The model under review builds one solid part; all positions refer to its coordinate system, in mm. A direction names the side the tool comes from. Round coordinates to 2 decimals unless told otherwise and drop trailing zeros. Loops run counter-clockwise (first coordinate to the right, second up) from the corner with the lowest first, then second, coordinate; pieces in that order, holes last. Notation, with made-up numbers: (31, 13) -> (39, 13) arc R32 ccw to (39, 45) -> close; hole circle Ø5 at (69.5, -14.75). An arc over 180 degrees is marked (long way). Write each question's results on one line, items separated by ' | '. Start each with the question number.
Item 1: We need section B-B (y = -12). Give the boundary of the cut face in (x, z), and give its area (3 significant figures).
Item 2: Clearance check with flat-ended pins moving along their axes: pin 1 Ø4 at (x, y) = (-13.5, -5) entering from +Z; pin 2 Ø5 at (y, z) = (-11.5, 12.5) entering from +X; pin 3 Ø6 at (x, y) = (-21.5, -3) entering from -Z; pin 4 Ø7.5 at (y, z) = (-6.5, 10.5) entering from -X. State where each tip first meets the part, or that it passes through.
Item 3: For L1, parallel to Y at x = 26.5, z = 4.8; L2, parallel to Z at x = 23.5, y = -4.25; L3, parallel to Y at x = -24, z = 4, list the stretches that pass through material, from the lowest coordinate up. Write a range as from..to.
Item 4: Tool access review of faces 1 (the flat face through (22.8, -7.1, 6)), 2 (the flat face through (0, -14.5, 10)): name each direction out of +Z, -Z, +X, -X, +Y, -Y from which nothing blocks a thin tool from reaching the whole face with its end or side.
Item 5: Mouldability with a two-part tool opening along Y and no side actions: class faces 3 (the cylindrical face through (23.267, -8.591, 2.958)), 4 (the flat face through (0, -7, 0)), 5 (the flat face through (0, 0, 10)) as pulls with the +Y half, pulls with the -Y half, needs draft (parallel to the pull), parting line crosses it, or undercut.
Item 6: We need section A-A (y = -7.25). Give the boundary of the cut face in (x, z), and give its area (3 significant figures).
Item 7: We need section D-D (z = 20). Give the boundary of the cut face in (x, y).
Item 8: We need section C-C (x = -26.5). Give the boundary of the cut face in (y, z).
from build123d import *

# Parameters (mm, degrees)
F1_DEPTH = 14.5
F3_DEPTH = 14.5
F4_R     = 1
F5_R     = 3.5
F6_DEPTH = 6


with BuildPart() as f1:
    # F0 (on Front) → F1 (new body)
    with BuildSketch(Plane.XZ):
        with BuildLine():
            Line((-33.5, 0), (-0.8672476206, 0))
            Line((-0.8672476206, 0), (0, 0))
            Line((0, 0), (0.8527118365, 0))
            Line((0.8527118365, 0), (33.5, 0))
            Line((33.5, 0), (33.5, 6))
            Line((33.5, 6), (17.4809702634, 6))
            Line((17.4809702634, 6), (17.4809702634, 16.8373537033))
            Line((17.4809702634, 16.8373537033), (17.4809702634, 18.120359887))
            ThreePointArc((17.4809702634, 18.120359887), (-0.8075640242, 34.9605479634), (-17.4809702634, 16.5198336275))
            Line((-17.4809702634, 16.5198336275), (-17.4809702634, 6))
            Line((-17.4809702634, 6), (-33.5, 6))
            Line((-33.5, 6), (-33.5, 0))
        make_face()
    extrude(amount=F1_DEPTH)

    # F2 (on face) → F3 (cut, through all)
    with BuildSketch(Plane.XZ.offset(14.5)):
        with BuildLine():
            ThreePointArc((0, 23), (-5, 18), (0, 13))
            Line((0, 13), (0, 23))
        make_face()
        with BuildLine():
            Line((0, 23), (0, 13))
            ThreePointArc((0, 13), (3.5355339059, 14.4644660941), (5, 18))
            ThreePointArc((5, 18), (3.5355339059, 21.5355339059), (0, 23))
        make_face()
    extrude(amount=-F3_DEPTH, mode=Mode.SUBTRACT)

    # F4
    f4_edges = [f1.edges().sort_by_distance(p)[0] for p in [
        (-17.48097, -7.25, 6),
        (17.48097, -7.25, 6),
    ]]
    fillet(f4_edges, radius=F4_R)

    # F5 (on face) → F6 (cut, through all)
    with BuildSketch(Plane(origin=(0, 0, 0), x_dir=(1, 0, 0), z_dir=(0, 0, -1))):
        with BuildLine():
            Line((23, 7.25), (30, 7.25))
            ThreePointArc((30, 7.25), (26.5, 10.75), (23, 7.25))
        make_face()
        with BuildLine():
            ThreePointArc((23, 7.25), (26.5, 3.75), (30, 7.25))
            Line((30, 7.25), (23, 7.25))
        make_face()
        with Locations((-26.5, 7.25)):
            Circle(F5_R)
    extrude(amount=-F6_DEPTH, mode=Mode.SUBTRACT)


solid = f1.part
Here are the results:
1) outline: (-33.5, 0) -> (33.5, 0) -> (33.5, 6) -> (18.48, 6) arc R1 cw to (17.48, 7) -> (17.48, 18.12) arc R17.5 ccw (long way) to (-17.48, 16.52) -> (-17.48, 7) arc R1 cw to (-18.48, 6) -> (-33.5, 6) -> close; hole circle Ø10 at (0, 18) | area: 1,210 mm2
2) pin 1: stops at z = 30.68 | pin 2: stops at x = 17.48 | pin 3: stops at z = 0 | pin 4: stops at x = -17.51
3) L1: y = -14.5..-10.75, -3.75..0 | L2: z = 0..6 | L3: y = -14.5..-9.7, -4.8..0
4) face 1: +Z, +X, +Y, -Y | face 2: +Z, -Z, +X, -X, -Y
5) face 3: undercut | face 4: needs draft | face 5: pulls with the +Y half
6) outline: (-33.5, 0) -> (-30, 0) -> (-30, 6) -> (-33.5, 6) -> close; (-23, 0) -> (23, 0) -> (23, 6) -> (18.48, 6) arc R1 cw to (17.48, 7) -> (17.48, 18.12) arc R17.5 ccw (long way) to (-17.48, 16.52) -> (-17.48, 7) arc R1 cw to (-18.48, 6) -> (-23, 6) -> close; (30, 0) -> (33.5, 0) -> (33.5, 6) -> (30, 6) -> close; hole circle Ø10 at (0, 18) | area: 1,120 mm2
7) outline: (-17.32, -14.5) -> (-4.58, -14.5) -> (-4.58, 0) -> (-17.32, 0) -> close; (4.58, -14.5) -> (17.31, -14.5) -> (17.31, 0) -> (4.58, 0) -> close
8) outline: (-14.5, 0) -> (-10.75, 0) -> (-10.75, 6) -> (-14.5, 6) -> close; (-3.75, 0) -> (0, 0) -> (0, 6) -> (-3.75, 6) -> close
